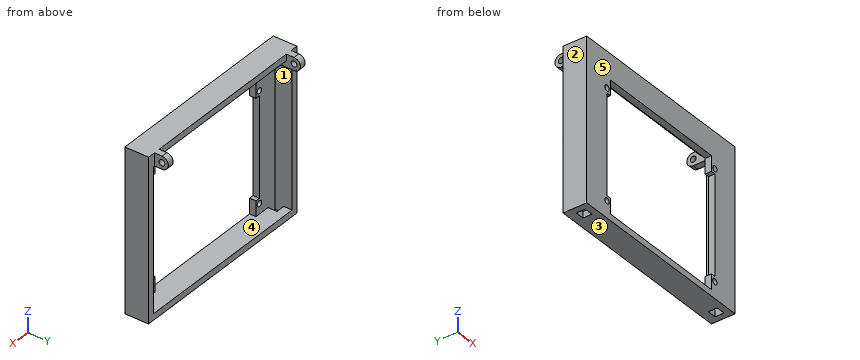
from build123d import *

# Parameters (mm, degrees)
SKETCH1_W           = 154
SKETCH1_H           = 127
SKETCH1_R           = 2.25
BOSS_EXTRUDE1_DEPTH = 5
SKETCH2_R           = 2.25
BOSS_EXTRUDE2_DEPTH = 11
SKETCH4_W           = 6
SKETCH4_H           = 10
CUT_EXTRUDE1_DEPTH  = 37
SKETCH5_W           = 132
SKETCH5_H           = 5
SKETCH5_W_2         = 1
SKETCH5_W_3         = 6
BOSS_EXTRUDE3_DEPTH = 13.65
SKETCH6_W           = 7
SKETCH6_H           = 7
CUT_EXTRUDE2_DEPTH  = 13.65


with BuildPart() as part:
    # Sketch1 → Boss-Extrude1 (new body)
    with BuildSketch(Plane(origin=(0, 0, 0), x_dir=(1, 0, 0), z_dir=(0, 1, 0))):
        with Locations((0, -7.5)):
            Rectangle(SKETCH1_W, SKETCH1_H)
        with Locations(Location((-56, -43, 0), (0, 0, 270))):
            Circle(SKETCH1_R, mode=Mode.SUBTRACT)
        with Locations(Location((56, -43, 0), (0, 0, 270))):
            Circle(SKETCH1_R, mode=Mode.SUBTRACT)
        with Locations(Location((-56, 43, 0), (0, 0, 270))):
            Circle(SKETCH1_R, mode=Mode.SUBTRACT)
        Polygon((52.5, -39), (52.5, -51), (-52.5, -51), (-52.5, -39), (-56, -39), (-56, 39), (-52.5, 39), (-52.5, 51), (52.5, 51), (52.5, 39), (56, 39), (56, -39), align=None, mode=Mode.SUBTRACT)
        with Locations(Location((56, 43, 0), (0, 0, 270))):
            Circle(SKETCH1_R, mode=Mode.SUBTRACT)
    extrude(amount=BOSS_EXTRUDE1_DEPTH)

    # Sketch2 → Boss-Extrude2 (add)
    with BuildSketch(Plane.ZY.offset(77)):
        with BuildLine():
            ThreePointArc((71, 24.65), (66, 29.65), (61, 24.65))
            Line((61, 24.65), (61, 5))
            Line((61, 5), (71, 5))
            Line((71, 5), (71, 24.65))
        make_face()
        with Locations((66, 24.65)):
            Circle(SKETCH2_R, mode=Mode.SUBTRACT)
    boss_extrude2 = extrude(amount=-BOSS_EXTRUDE2_DEPTH)

    # Sketch4 → Cut-Extrude1 (cut)
    with BuildSketch(Plane(origin=(0, 5, 0), x_dir=(1, 0, 0), z_dir=(0, 1, 0))):
        with Locations((-74, -66)):
            Rectangle(SKETCH4_W, SKETCH4_H)
    cut_extrude1 = extrude(amount=CUT_EXTRUDE1_DEPTH, mode=Mode.SUBTRACT)

    # Mirror1: Boss-Extrude2, Cut-Extrude1 across plane
    add(boss_extrude2.mirror(Plane(origin=(0, 0, 0), x_dir=(0, 0, 1), z_dir=(1, 0, 0))))
    add(cut_extrude1.mirror(Plane(origin=(0, 0, 0), x_dir=(0, 0, 1), z_dir=(1, 0, 0))), mode=Mode.SUBTRACT)

    # Sketch5 → Boss-Extrude3 (add)
    with BuildSketch(Plane(origin=(0, 5, 0), x_dir=(1, 0, 0), z_dir=(0, 1, 0))):
        Polygon((71, -71), (77, -71), (77, 56), (-77, 56), (-77, -71), (-71, -71), (-71, -66), (-72, -66), (-72, -61), (-72, 51), (-52.5, 51), (52.5, 51), (72, 51), (72, -61), (72, -66), (71, -66), align=None)
        with Locations((0, -68.5)):
            Rectangle(SKETCH5_W, SKETCH5_H)
        with Locations((71.5, -63.5)):
            Rectangle(SKETCH5_W_2, SKETCH5_H)
        with Locations((-69, -63.5)):
            Rectangle(SKETCH5_W_3, SKETCH5_H)
    extrude(amount=BOSS_EXTRUDE3_DEPTH)

    # Sketch6 → Cut-Extrude2 (cut)
    with BuildSketch(Plane.XY.offset(-51)):
        with Locations((68.5, 8.5)):
            Rectangle(SKETCH6_W, SKETCH6_H)
    cut_extrude2 = extrude(amount=-CUT_EXTRUDE2_DEPTH, mode=Mode.SUBTRACT)

    # Mirror2: Cut-Extrude2 across plane
    add(cut_extrude2.mirror(Plane(origin=(0, 0, 0), x_dir=(0, 0, 1), z_dir=(1, 0, 0))), mode=Mode.SUBTRACT)


solid = part.part
Verification items for the finished model (mm, model axes). Face numbers are marked on the shaded views. A direction names the side the tool comes from. Give positions to 0.01 mm unless a question says otherwise; leave off trailing zeros. Write each loop counter-clockwise with the first axis right and the second up, starting at its lowest first coordinate (ties: lowest second). Pieces come first, ordered by that corner, then holes.
(1) Mould release check, pull along X, two halves, no side actions. Record for the marked faces 1, 2 and 3: +X half, -X half, draft (parallel to the pull), parting line (faces both ways), or undercut.
(2) Cross-section at A-A (z = -7.5). Enter the section's corners in (x, y), plus the area to 4 significant figures.
(3) Access from +Z, -Z, +X, -X, +Y, -Y to the whole of each face (thin tool, end or side, straight path). Record for the marked faces 4 and 5.
(4) Material ranges on line 1 (X direction, y = 3.1, z = 43); line 2 (Z direction, x = 55, y = 9.75); line 3 (X direction, y = 1.75, z = 33), recorded low to high.
(5) Cross-section at B-B (y = 7.5). Enter the section's corners in (x, z), plus the area to 3 significant figures.
(6) Cross-section at D-D (x = -40). Enter the section's corners in (y, z).
(7) Gauge pin test, flat ends, axial feed: pin 1 (4 mm diameter, centred on x = -56, z = 43, fed in from +Y); pin 2 (5.5 mm diameter, centred on x = 9, z = 69.5, fed in from +Y); pin 3 (8 mm diameter, centred on y = 25, z = 66, fed in from +X). Record the tip position at first contact, or that the pin passes through.
(8) Cross-section at C-C (z = -43). Enter the section's corners in (x, y), plus the area to 4 significant figures.
Worked out:
1. face 1: undercut
1. face 2: -X half
1. face 3: draft
2. outline: (-77, 0) - (-56, 0) - (-56, 5) - (-72, 5) - (-72, 18.65) - (-77, 18.65) - close; (56, 0) - (77, 0) - (77, 18.65) - (72, 18.65) - (72, 5) - (56, 5) - close
2. area: 346.5 mm2
3. face 4: +Y
3. face 5: +Z, -Z, +X, -X, -Y
4. line 1: x = -77 to -58.25, -53.75 to -52.5, 52.5 to 53.75, 58.25 to 77
4. line 2: z = -56 to -51, 66 to 71
4. line 3: x = -77 to -56, 56 to 77
5. outline: (-77, -56) - (-72, -56) - (-72, 61) - (-66, 61) - (-66, 66) - (66, 66) - (66, 61) - (72, 61) - (72, -56) - (77, -56) - (77, 71) - (-77, 71) - close; (-65, -56) - (65, -56) - (65, -51) - (-65, -51) - close
5. area: 2,700 mm2
6. outline: (0, -56) - (18.65, -56) - (18.65, -51) - (0, -51) - close; (0, 51) - (5, 51) - (5, 66) - (18.65, 66) - (18.65, 71) - (0, 71) - close
7. pin 1: passes through
7. pin 2: stops at y = 18.65
7. pin 3: stops at x = 71
8. outline: (-77, 0) - (-58.25, 0) - (-58.25, 5) - (-72, 5) - (-72, 18.65) - (-77, 18.65) - close; (-53.75, 0) - (-52.5, 0) - (-52.5, 5) - (-53.75, 5) - close; (52.5, 0) - (53.75, 0) - (53.75, 5) - (52.5, 5) - close; (58.25, 0) - (77, 0) - (77, 18.65) - (72, 18.65) - (72, 5) - (58.25, 5) - close
8. area: 336.5 mm2
